Can you work these out from the model? Positions are in its coordinate system, mm. Face numbers are marked on the shaded views. A direction names the side the tool comes from. Give positions to 0.01 mm unless a question says otherwise; leave off trailing zeros. Write each loop counter-clockwise with the first axis right and the second up, starting at its lowest first coordinate (ties: lowest second). Pieces come first, ordered by that corner, then holes.
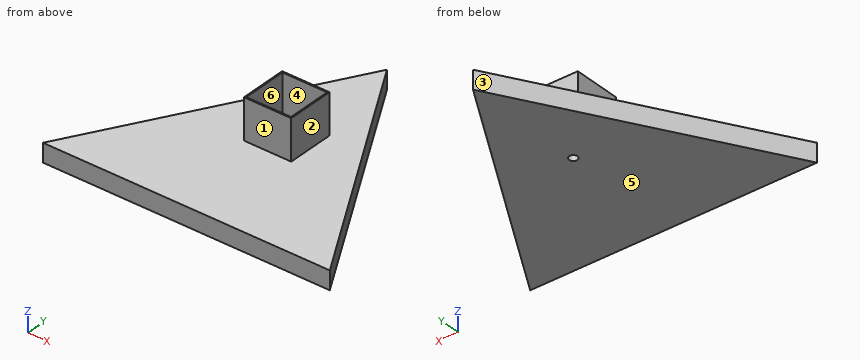
from build123d import *

# Parameters (mm, degrees)
F1_DEPTH = 11
F3_W     = 28
F3_H     = 28
F4_DEPTH = 24
F2_W     = 26.5
F2_H     = 26.5
F5_DEPTH = 24
F6_R     = 2.5
F7_DEPTH = 25


with BuildPart() as f1:
    # F0 (on Top) → F1 (new body)
    with BuildSketch(Plane.XY):
        Polygon((0, 73.612159), (-85, -73.612159), (0, -73.612159), align=None)
        Polygon((0, 73.612159), (0, -73.612159), (85, -73.612159), align=None)
    extrude(amount=F1_DEPTH)

    # F3 (on face) → F4 (join)
    with BuildSketch(Plane.XY.offset(11)):
        Rectangle(F3_W, F3_H)
    extrude(amount=F4_DEPTH)

    # F2 (on face) → F5 (cut)
    with BuildSketch(Plane.XY.offset(11)):
        Rectangle(F2_W, F2_H)
    extrude(amount=F5_DEPTH, mode=Mode.SUBTRACT)

    # F6 (on face) → F7 (cut)
    with BuildSketch(Plane.XY.offset(11)):
        Circle(F6_R)
    extrude(amount=-F7_DEPTH, mode=Mode.SUBTRACT)


solid = f1.part
(1) Imagine slicing it at C-C, the plane x = 42.5. Write out the boundary of the cut face in (y, z).
Returned:
outline: (-73.61, 0) - (0, 0) - (0, 11) - (-73.61, 11) - close
(2) Imagine slicing it at D-D, the plane z = 2. Write out the boundary of the cut face in (x, y), plus the area to 3 significant figures.
Returned:
outline: (-85, -73.61) - (85, -73.61) - (0, 73.61) - close; hole circle Ø5 at (0, 0)
area: 12,500 mm2
(3) If I drill on L1, parallel to Y at x = 12, z = 31.5; L2, parallel to Y at x = 0, z = 7; L3, parallel to Z at x = 48, y = -21.5, over which ranges is the centre line in solid material (lowest first)?
Returned:
L1: y = -14 to -13.25, 13.25 to 14
L2: y = -73.61 to -2.5, 2.5 to 73.61
L3: z = 0 to 11
(4) Imagine slicing it at B-B, the plane y = 0. Write out the boundary of the cut face in (x, z).
Returned:
outline: (-42.5, 0) - (-2.5, 0) - (-2.5, 11) - (-13.25, 11) - (-13.25, 35) - (-14, 35) - (-14, 11) - (-42.5, 11) - close; (2.5, 0) - (42.5, 0) - (42.5, 11) - (14, 11) - (14, 35) - (13.25, 35) - (13.25, 11) - (2.5, 11) - close
(5) Will these pins go through, and if not, where does the flat tip stop? P1, Ø6, axis at x = 31, y = 11, coming from the +Z side; P2, Ø21, axis at x = -4.5, y = -1.5, coming from the +Z side; P3, Ø12, axis at y = 3.5, z = 20.5, coming from the -X side; P4, Ø12, axis at x = 26.5, z = 5.5, coming from the +Y side.
Returned:
P1: stops at z = 11
P2: stops at z = 35
P3: stops at x = -14
P4: stops at y = 38.11
(6) If we mould it in two halves opening along Y, with no side actions, what happens to the marked faces 1, 2, 3 and 4? For each: +Y half, -Y half, draft (parallel to the pull), parting line (faces both ways), or undercut.
Returned:
face 1: -Y half
face 2: draft
face 3: +Y half
face 4: undercut
(7) Imagine slicing it at A-A, the plane z = 27.5. Write out the boundary of the cut face in (x, y).
Returned:
outline: (-14, -14) - (14, -14) - (14, 14) - (-14, 14) - close; hole (-13.25, -13.25) - (13.25, -13.25) - (13.25, 13.25) - (-13.25, 13.25) - close
(8) For the marked faces 5 and 6, which set-ups out of +Z, -Z, +X, -X, +Y, -Y let a thin tool reach every point of the face, with its end or its side?
Returned:
face 5: -Z, +X, -X, +Y, -Y
face 6: +Z
